Check sheet for the drawn part. Datum: minimum x, y, z corner. Units: mm. A direction names the side the tool comes from. Round coordinates to 2 decimals unless told otherwise and drop trailing zeros. Write each loop counter-clockwise with the first axis right and the second up, starting at its lowest first coordinate (ties: lowest second). Pieces come first, ordered by that corner, then holes.
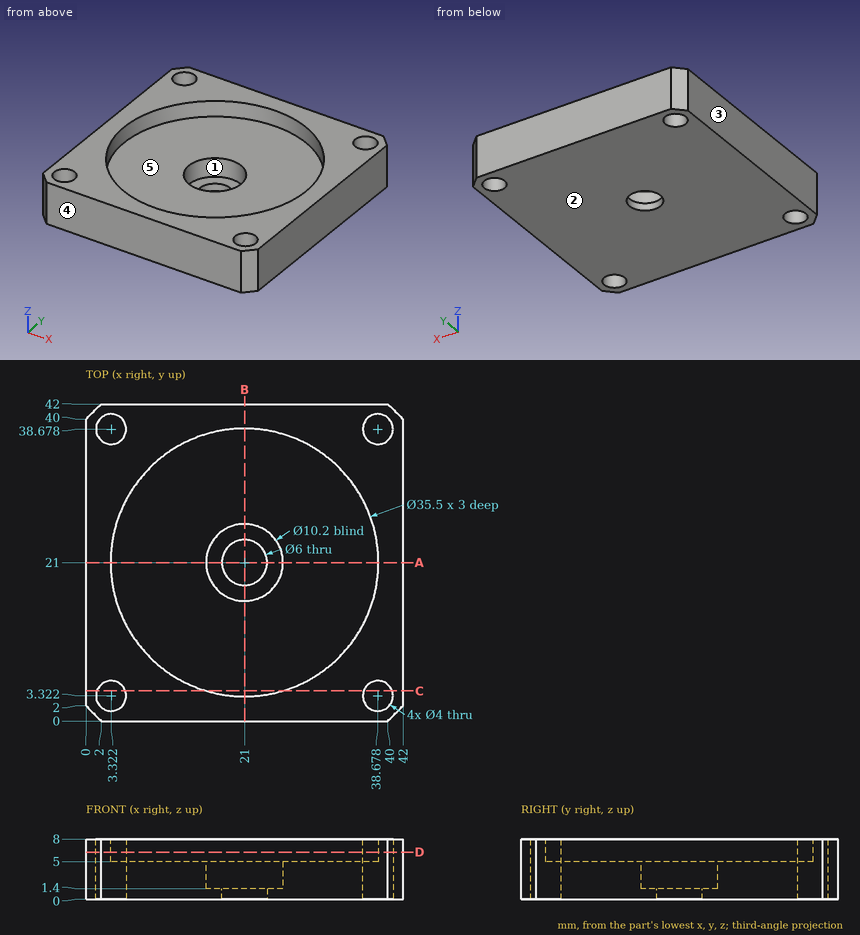
Q1. Tool access check on the marked faces 1 and 2. Record the directions out of +Z, -Z, +X, -X, +Y, -Y that give a thin tool (end or side, any length) a straight path to the whole face; none if there is none.
Recorded:
face 1: +Z
face 2: -Z, +X, -X, +Y, -Y
Q2. Material ranges on line 1 along Y through (x, z) = (21, 5.9); line 2 along X through (y, z) = (5, 5.5) (1 decimal); line 3 along Y through (x, z) = (21, 2.4), recorded low to high.
Recorded:
line 1: y = 0 to 3.25, 38.75 to 42
line 2: x = 0 to 2.2, 4.4 to 13.3, 28.7 to 37.6, 39.8 to 42
line 3: y = 0 to 15.9, 26.1 to 42
Q3. Sectioned sample at C-C (y = 4). Enter the section's corners in (x, z) (1 decimal), plus the area to 3 significant figures.
Recorded:
outline: (0, 0) - (1.4, 0) - (1.4, 8) - (0, 8) - close; (5.2, 0) - (36.8, 0) - (36.8, 8) - (26.1, 8) - (26.1, 5) - (15.9, 5) - (15.9, 8) - (5.2, 8) - close; (40.6, 0) - (42, 0) - (42, 8) - (40.6, 8) - close
area: 245 mm2
Q4. Depth check by flat-ended pin: P1, Ø8, axis at x = 19.5, y = 23, coming from the +Z side; P2, Ø2.5, axis at x = 38.68, y = 3.32, coming from the -Z side. Enter the tip coordinate at first touch or a pass-through.
Recorded:
P1: stops at z = 5
P2: passes through
Q5. Sectioned sample at A-A (y = 21). Enter the section's corners in (x, z).
Recorded:
outline: (0, 0) - (18, 0) - (18, 1.4) - (15.9, 1.4) - (15.9, 5) - (3.25, 5) - (3.25, 8) - (0, 8) - close; (24, 0) - (42, 0) - (42, 8) - (38.75, 8) - (38.75, 5) - (26.1, 5) - (26.1, 1.4) - (24, 1.4) - close
Q6. Sectioned sample at D-D (z = 6.25). Enter the section's corners in (x, y).
Recorded:
outline: (0, 2) - (2, 0) - (40, 0) - (42, 2) - (42, 40) - (40, 42) - (2, 42) - (0, 40) - close; hole circle Ø4 at (3.32, 3.32); hole circle Ø4 at (3.32, 38.68); hole circle Ø35.5 at (21, 21); hole circle Ø4 at (38.68, 3.32); hole circle Ø4 at (38.68, 38.68)
Q7. Release check for a two-part mould opening along Y. For the marked faces 3, 4 and 5 record: released by +Y, released by -Y, zero draft, split by the parting line, or undercut.
Recorded:
face 3: zero draft
face 4: released by -Y
face 5: undercut
